The listing builds one solid part. Answer for the finished solid, in the listing's coordinates (mm). A direction names the side the tool comes from. Coordinates: 2 decimals unless noted, no trailing zeros. Write each loop counter-clockwise with the first axis right and the second up, starting at its lowest first coordinate (ties: lowest second). Pieces come first, ordered by that corner, then holes.
from build123d import *

# Parameters (mm, degrees)
BOSS_EXTRUDE1_DEPTH      = 152.4
BOSS_EXTRUDE1_DEPTH_BACK = 76.2
SKETCH1_W                = 76.2
SKETCH1_H                = 50.8
SKETCH1_W_2              = 63.5
SKETCH1_H_2              = 38.1
CUT_EXTRUDE1_DEPTH       = 804.658803572
CUT_EXTRUDE1_DEPTH_BACK  = 804.658803572
SKETCH2_R                = 2.6035
SKETCH2_R_2              = 2.603499999
SKETCH3_R                = 2.6035
CUT_EXTRUDE2_DEPTH       = 807.363629238
SKETCH4_R                = 2.6035
CUT_EXTRUDE3_DEPTH       = 166.1
CUT_EXTRUDE4_REACH       = 167.1
SKETCH5_R                = 2.6035


with BuildPart() as part:
    # Sketch1 → Boss-Extrude1 (new, two sides: drawn at the far end of the back side and taken through both)
    with BuildSketch(Plane.XY.offset(-BOSS_EXTRUDE1_DEPTH_BACK)):
        with Locations((0, 762.756140976)):
            Rectangle(SKETCH1_W, SKETCH1_H)
        with Locations((0, 762.756140976)):
            Rectangle(SKETCH1_W_2, SKETCH1_H_2, mode=Mode.SUBTRACT)
    extrude(amount=BOSS_EXTRUDE1_DEPTH + BOSS_EXTRUDE1_DEPTH_BACK)

    # Sketch2 → Cut-Extrude1 (cut, two sides: drawn at the far end of the back side and taken through both)
    with BuildSketch(Plane(origin=(0, 0, 0), x_dir=(0, 0, -1), z_dir=(1, 0, 0)).offset(-CUT_EXTRUDE1_DEPTH_BACK)):
        with Locations((62.346011746, 750.056140976)):
            Circle(SKETCH2_R)
        with Locations(Location((34.638035237, 750.056140976, 0), (0, 0, 90))):
            Circle(SKETCH2_R)
        with Locations((34.638035237, 775.456140976)):
            Circle(SKETCH2_R)
        with Locations(Location((62.346011746, 775.456140976, 0), (0, 0, 90))):
            Circle(SKETCH2_R)
        with Locations((11.259046982, 750.056140976)):
            Circle(SKETCH2_R_2)
        with Locations((11.259046982, 775.456140976)):
            Circle(SKETCH2_R_2)
        with Locations((-17.315953018, 762.756140976)):
            Circle(SKETCH2_R_2)
        with Locations((-45.890953018, 775.456140976)):
            Circle(SKETCH2_R_2)
        with Locations((-45.890953018, 750.056140976)):
            Circle(SKETCH2_R_2)
    extrude(amount=CUT_EXTRUDE1_DEPTH + CUT_EXTRUDE1_DEPTH_BACK, mode=Mode.SUBTRACT)

    # Sketch3 → Cut-Extrude2 (cut, through all)
    with BuildSketch(Plane(origin=(38.1, 0, 0), x_dir=(0, 0, -1), z_dir=(1, 0, 0))):
        with Locations((-134.9375, 769.106140976)):
            Circle(SKETCH3_R)
        with Locations((-134.9375, 756.406140976)):
            Circle(SKETCH3_R)
    extrude(amount=-CUT_EXTRUDE2_DEPTH, mode=Mode.SUBTRACT)

    # Sketch4 → Cut-Extrude3 (cut, through all)
    with BuildSketch(Plane(origin=(0, 788.156140976, 0), x_dir=(1, 0, 0), z_dir=(0, 1, 0))):
        with Locations(Location((20.32, 58.7375, 0), (0, 0, 270))):
            Circle(SKETCH4_R)
        with Locations(Location((-20.32, 58.7375, 0), (0, 0, 270))):
            Circle(SKETCH4_R)
    extrude(amount=-CUT_EXTRUDE3_DEPTH, mode=Mode.SUBTRACT)

    # Sketch5 → Cut-Extrude4 (cut, up to next)
    with BuildSketch(Plane.XZ.offset(-737.356140976), mode=Mode.PRIVATE) as cut_extrude4_sk1:
        with Locations(Location((0, 138.1125, 0), (0, 0, 270))):
            Circle(SKETCH5_R)
    cut_extrude4_tool1 = extrude(cut_extrude4_sk1.sketch, amount=-CUT_EXTRUDE4_REACH, mode=Mode.PRIVATE) & part.part
    # Sketch5 → Cut-Extrude4 (cut, up to next)
    with BuildSketch(Plane.XZ.offset(-737.356140976), mode=Mode.PRIVATE) as cut_extrude4_sk2:
        with Locations(Location((0, 122.2375, 0), (0, 0, 270))):
            Circle(SKETCH5_R)
    cut_extrude4_tool2 = extrude(cut_extrude4_sk2.sketch, amount=-CUT_EXTRUDE4_REACH, mode=Mode.PRIVATE) & part.part
    add(cut_extrude4_tool1.solids().sort_by_distance((0, 737.356141, 138.1125))[0], mode=Mode.SUBTRACT)
    add(cut_extrude4_tool2.solids().sort_by_distance((0, 737.356141, 122.2375))[0], mode=Mode.SUBTRACT)


solid = part.part
Q1. Determine the mould class of faces 4 (the face through (34.881, 752.637, -62.007)), 5 (the face through (-21.904, 740.576, -60.804)), 6 (the face through (-38.1, 762, 36)) for opening direction X: released by +X, released by -X, zero draft, split by the parting line, or undercut.
Answers below:
face 4: zero draft
face 5: undercut
face 6: released by -X
Q2. Find the intervals of material crossed by probe 1 along X at (y, z) = (778.5, 140); probe 2 along Z at (x, y) = (32.5, 762.5), in increasing order.
Answers below:
probe 1: x = -38.1 to -31.75, 31.75 to 38.1
probe 2: z = -76.2 to 14.73, 19.91 to 152.4
Q3. The part is cut by section C-C, the plane z = -41. Write down the section's boundary in (x, y), then the cut area to 3 significant figures.
Answers below:
outline: (-38.1, 737.36) - (38.1, 737.36) - (38.1, 788.16) - (-38.1, 788.16) - close; hole (-31.75, 743.71) - (31.75, 743.71) - (31.75, 781.81) - (-31.75, 781.81) - close
area: 1,450 mm2
Q4. Which of the six approach directions +Z, -Z, +X, -X, +Y, -Y give full straight-line access (tool end or side, diameter ignored) to faces 1 (the face through (38.1, 762, 36)), 2 (the face through (0.782, 740.487, 119.754)), 3 (the face through (0, 781.806, 36))?
Answers below:
face 1: +Z, -Z, +X, +Y, -Y
face 2: -Y
face 3: +Z, -Z
Q5. The part is cut by section B-B, the plane x = 25. Write down the section's boundary in (y, z), then the cut area to 3 significant figures.
Answers below:
outline: (737.36, -76.2) - (743.71, -76.2) - (743.71, 152.4) - (737.36, 152.4) - close; (781.81, -76.2) - (788.16, -76.2) - (788.16, 152.4) - (781.81, 152.4) - close
area: 2,900 mm2
Q6. The part is cut by section A-A, the plane x = -20.32. Write down the section's boundary in (y, z).
Answers below:
outline: (737.36, -76.2) - (743.71, -76.2) - (743.71, -61.34) - (737.36, -61.34) - close; (737.36, -56.13) - (743.71, -56.13) - (743.71, 152.4) - (737.36, 152.4) - close; (781.81, -76.2) - (788.16, -76.2) - (788.16, -61.34) - (781.81, -61.34) - close; (781.81, -56.13) - (788.16, -56.13) - (788.16, 152.4) - (781.81, 152.4) - close
Q7. Given pin 1 (4.5 mm diameter, centred on x = -20.32, z = -58.74, fed in from -Y); pin 2 (3 mm diameter, centred on x = 0, z = 138.11, fed in from -Y), each flat-ended and moving along its own axis, determine where each tip first touches the part or whether it passes through.
Answers below:
pin 1: passes through
pin 2: stops at y = 781.81
